from build123d import *

# Parameters (mm, degrees)
F0_W      = 60
F0_H      = 81
F1_DEPTH  = 1.5
F2_R      = 1.5
F3_DEPTH  = 1.501
F4_W      = 7.6
F4_H      = 5.8
F5_DEPTH  = 16.5
F6_W      = 5
F6_H      = 13.6
F6_W_2    = 6.05
F6_H_2    = 18
F7_DEPTH  = 8
F8_R      = 3.15
F8_W      = 6.3
F8_H      = 6.3
F9_DEPTH  = 9.5
F10_R     = 2.675
F11_DEPTH = 3.5
F12_R     = 3.85
F12_R_2   = 3.15
F13_DEPTH = 5
F14_R     = 3.85
F15_DEPTH = 3


with BuildPart() as f1:
    # F0 (on Top) → F1 (new body)
    with BuildSketch(Plane.XY):
        Rectangle(F0_W, F0_H)
    extrude(amount=F1_DEPTH)

    # F2 (on face) → F3 (cut, through all)
    with BuildSketch(Plane.XY.offset(1.5)):
        with Locations((-27, -37.5)):
            Circle(F2_R)
        with Locations((-27, -7.5)):
            Circle(F2_R)
        with Locations((-27, 18.5)):
            Circle(F2_R)
        with Locations((27, 18.5)):
            Circle(F2_R)
        with Locations((27, -7.5)):
            Circle(F2_R)
        with Locations((27, -37.5)):
            Circle(F2_R)
    extrude(amount=-F3_DEPTH, mode=Mode.SUBTRACT)

    # F4 (on face) → F5 (join)
    with BuildSketch(Plane.XY.offset(1.5)):
        with Locations((8.35, 7.9)):
            Rectangle(F4_W, F4_H)
        with Locations((21.95, 7.9)):
            Rectangle(F4_W, F4_H)
    extrude(amount=F5_DEPTH)

    # F6 (on face) → F7 (join)
    with BuildSketch(Plane.XY.offset(1.5)):
        with Locations((2, 39.7)):
            Rectangle(F6_W, F6_H)
        with Locations((-11, 39.7)):
            Rectangle(F6_W, F6_H)
        with Locations((-23, 37.5)):
            Rectangle(F6_W_2, F6_H_2)
    extrude(amount=F7_DEPTH)

    # F8 (on face) → F9 (join)
    with BuildSketch(Plane(origin=(0, 0, 0), x_dir=(1, 0, 0), z_dir=(0, 0, -1))):
        with Locations((-25, 23.5)):
            Circle(F8_R)
        with Locations((0, 23.5)):
            Rectangle(F8_W, F8_H)
        with Locations((25, 23.5)):
            Rectangle(F8_W, F8_H)
    extrude(amount=F9_DEPTH)

    # F10 (on face) → F11 (join)
    with BuildSketch(Plane(origin=(0, 0, 0), x_dir=(1, 0, 0), z_dir=(0, 0, -1))):
        with Locations((12.4, 15.5)):
            Circle(F10_R)
        with Locations((-12.4, 15.5)):
            Circle(F10_R)
    extrude(amount=F11_DEPTH)

    # F12 (on face) → F13 (join)
    with BuildSketch(Plane(origin=(0, 0, -9.5), x_dir=(1, 0, 0), z_dir=(0, 0, -1))):
        with Locations((-25, 23.5)):
            Circle(F12_R)
        with Locations((-25, 23.5)):
            Circle(F12_R_2, mode=Mode.SUBTRACT)
        with Locations((-25, 23.5)):
            Circle(F12_R_2)
    extrude(amount=-F13_DEPTH)

    # F14 (on face) → F15 (join)
    with BuildSketch(Plane(origin=(0, 0, -9.5), x_dir=(1, 0, 0), z_dir=(0, 0, -1))):
        Polygon((-27.280534, 19.55), (-22.719466, 19.55), (-20.438933, 23.5), (-22.719466, 27.45), (-27.280534, 27.45), (-29.561067, 23.5), align=None)
        with Locations((-25, 23.5)):
            Circle(F14_R, mode=Mode.SUBTRACT)
        with Locations((-25, 23.5)):
            Circle(F14_R)
    extrude(amount=-F15_DEPTH)


solid = f1.part
Part model, mm, in its own coordinate system. A direction names the side the tool comes from. Give positions to 0.01 mm unless a question says otherwise; leave off trailing zeros. Write each loop counter-clockwise with the first axis right and the second up, starting at its lowest first coordinate (ties: lowest second). Pieces come first, ordered by that corner, then holes.
1) Probe L1, parallel to Y at x = -27, z = 0.8; L2, parallel to Z at x = 12, y = 22.5; L3, parallel to Y at x = 27.5, z = -8.5. List the from-to ranges inside material, lowest first.
Resolved:
L1: y = -40.5 to -39, -36 to -9, -6 to 17, 20 to 40.5
L2: z = 0 to 1.5
L3: y = -26.65 to -20.35
2) Cut at B-B on y = 18.5. Write the cut outline in (x, z), then the cut area to 3 significant figures.
Resolved:
outline: (-30, 0) - (-28.5, 0) - (-28.5, 1.5) - (-30, 1.5) - close; (-25.5, 0) - (25.5, 0) - (25.5, 1.5) - (-25.5, 1.5) - close; (28.5, 0) - (30, 0) - (30, 1.5) - (28.5, 1.5) - close
area: 81.0 mm2
3) Two-plate mould, pull along Y, no slides. Class faces 6 (the face through (25.8, -38.4, 0.8)), 7 (the face through (8, 5, 10)), 8 (the face through (-28.437, -21.553, -8.021)), 9 (the face through (25.5, -7.43, 0.76)): released by +Y, released by -Y, zero draft, split by the parting line, or undercut.
Resolved:
face 6: undercut
face 7: released by -Y
face 8: released by +Y
face 9: undercut
4) Cut at D-D on z = 8.5. Write the cut outline in (x, y) (3 decimals), then the cut area to 3 significant figures.
Resolved:
outline: (-26.025, 28.5) - (-19.975, 28.5) - (-19.975, 46.5) - (-26.025, 46.5) - close; (-13.5, 32.9) - (-8.5, 32.9) - (-8.5, 46.5) - (-13.5, 46.5) - close; (-0.5, 32.9) - (4.5, 32.9) - (4.5, 46.5) - (-0.5, 46.5) - close; (4.55, 5) - (12.15, 5) - (12.15, 10.8) - (4.55, 10.8) - close; (18.15, 5) - (25.75, 5) - (25.75, 10.8) - (18.15, 10.8) - close
area: 333 mm2
5) Which spindle directions (+Z, -Z, +X, -X, +Y, -Y) get a long thin tool onto all of the face, cutting with end or side? Do faces 1 (the face through (21.85, -23, -5)), 2 (the face through (-21.595, -21.497, -8.021)), 3 (the face through (-24, -20, -4.5)), 4 (the face through (2, 32.9, 5)), 5 (the face through (0, -26.65, -5)). Say none if no direction does.
Resolved:
face 1: -Z, +Y, -Y
face 2: -Z, +Y
face 3: none
face 4: +Z, +X, -Y
face 5: -Z, +X, -Y
6) Pin check, flat tips, straight feed: pin 1 (6 mm diameter, centred on x = 16, y = 2.5, fed in from +Z); pin 2 (5 mm diameter, centred on x = -23, z = 1, fed in from +Y); pin 3 (3 mm diameter, centred on x = -13.5, y = 5.5, fed in from -Z); pin 4 (3 mm diameter, centred on x = 4, z = -5.5, fed in from +Y). Stop position of each tip, or through.
Resolved:
pin 1: stops at z = 1.5
pin 2: stops at y = 46.5
pin 3: stops at z = 0
pin 4: stops at y = -20.35
7) Cut at C-C on x = 8.5. Write the cut outline in (y, z).
Resolved:
outline: (-40.5, 0) - (40.5, 0) - (40.5, 1.5) - (10.8, 1.5) - (10.8, 18) - (5, 18) - (5, 1.5) - (-40.5, 1.5) - close
8) Cut at A-A on z = 13.75. Write the cut outline in (x, y), then the cut area to 3 significant figures.
Resolved:
outline: (4.55, 5) - (12.15, 5) - (12.15, 10.8) - (4.55, 10.8) - close; (18.15, 5) - (25.75, 5) - (25.75, 10.8) - (18.15, 10.8) - close
area: 88.2 mm2
